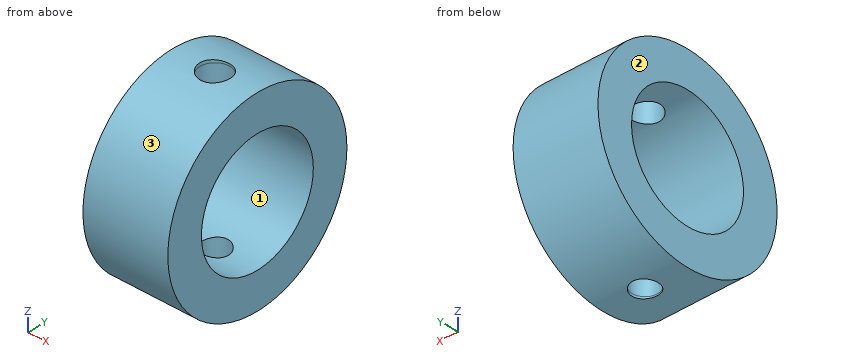
```python
from build123d import *

# Parameters (mm, degrees)
F2_R     = 12.7
F2_R_2   = 7.9375
F0_DEPTH = 5.55625


with BuildPart() as f0:
    # F2 (on Right) → F0 (new body, symmetric)
    with BuildSketch(Plane.YZ):
        Circle(F2_R)
        Circle(F2_R_2, mode=Mode.SUBTRACT)
    extrude(amount=F0_DEPTH, both=True)

    # F1 (on Front) → F3 (revolve, cut)
    with BuildSketch(Plane.XZ):
        Polygon((1.7145, -12.386102), (1.9812, 12.275856), (1.985787, 12.7), (0, 12.7), (0, -12.7), (1.711105, -12.7), align=None)
    revolve(axis=Axis((0, 0, 0), (0, 0, -1)), mode=Mode.SUBTRACT)


solid = f0.part
```
Part model, mm, in its own coordinate system. Face numbers are marked on the shaded views. Coordinates: 2 decimals unless noted, no trailing zeros. Order: outer loops, then holes, each group sorted by start corner. A loop starts at its lowest first (then second) coordinate and runs counter-clockwise, first axis right, second up. Notation, with made-up numbers: (27.25, -12) - (61.25, -12) arc R5 ccw to (61.25, -6) - close; hole circle Ø9 at (-5.5, -21). An arc over 180 degrees is marked (long way). Return JSON: item names as keys, results as strings. Group by question number.
Item 1: Pull direction Z, two halves, no side cores. Call the marked faces 1, 2 and 3: pulls with the +Z half, pulls with the -Z half, needs draft (parallel to the pull), parting line crosses it, or undercut.
Item 2: Pin check, flat tips, straight feed: pin 1 (4 mm diameter, centred on x = 2, z = -6, fed in from +Y); pin 2 (1 mm diameter, centred on x = -3, z = -7, fed in from -Y); pin 3 (6 mm diameter, centred on x = -2, y = -8, fed in from +Z). Stop position of each tip, or through.
Item 3: Cut at D-D (x = -3). List the corners of the cut face in (y, z) (1 decimal).
Item 4: Cut at B-B (y = 4.25). List the corners of the cut face in (x, z), plus the area to 3 significant figures.
Item 5: Cut at A-A (z = 0). List the corners of the cut face in (x, y).
Item 6: Drill centre lines: probe 1 along Z at (x, y) = (-3, 0); probe 2 along Z at (x, y) = (3.75, 2.75); probe 3 along Y at (x, z) = (-1, 2). Where is each one in solid material? Low to high. Write a range as from..to.
Item 7: Cut at C-C (z = -11). List the corners of the cut face in (x, y), plus the area to 3 significant figures.
Check values:
{
 "1": {"face 1": "undercut", "face 2": "needs draft", "face 3": "parting line crosses it"},
 "2": {"pin 1": "stops at y = 12.05", "pin 2": "stops at y = -10.91", "pin 3": "stops at z = 11.67"},
 "3": {"outline": "circle Ø25.4 at (0, 0); hole circle Ø15.9 at (0, 0)"},
 "4": {"outline": "(-5.56, -11.97) - (5.56, -11.97) - (5.56, -6.7) - (-5.56, -6.7) - close; (-5.56, 6.7) - (5.56, 6.7) - (5.56, 11.97) - (-5.56, 11.97) - close", "area": "117 mm2"},
 "5": {"outline": "(-5.56, -12.7) - (5.56, -12.7) - (5.56, -7.94) - (-5.56, -7.94) - close; (-5.56, 7.94) - (5.56, 7.94) - (5.56, 12.7) - (-5.56, 12.7) - close"},
 "6": {"probe 1": "z = -12.7..-7.94, 7.94..12.7", "probe 2": "z = -12.4..-7.45, 7.45..12.4", "probe 3": "y = -12.54..-7.68, 7.68..12.54"},
 "7": {"outline": "(-5.56, -6.35) - (5.56, -6.35) - (5.56, 6.35) - (-5.56, 6.35) - close; hole circle Ø3.46 at (0, 0)", "area": "132 mm2"}
}
